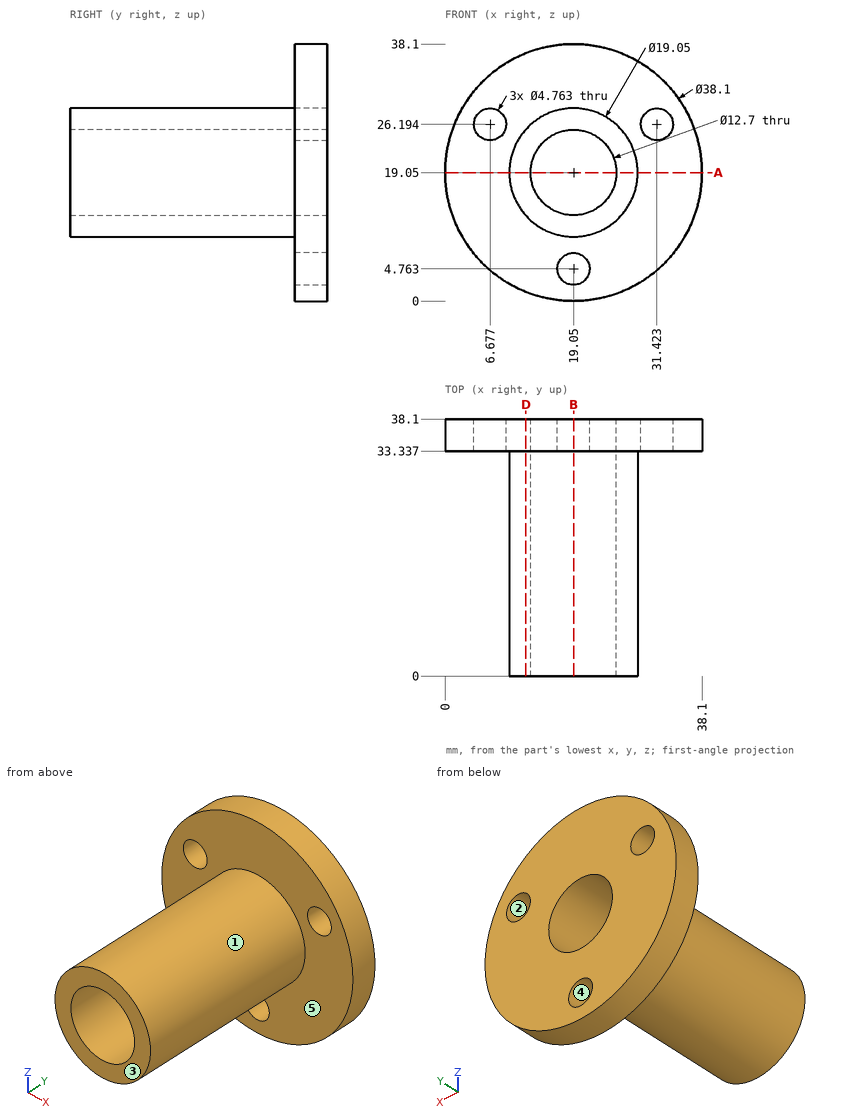
The drawing under review shows one solid part. Ordinate dimensions are in mm from its lowest x, y, z. A direction names the side the tool comes from. Give positions to 0.01 mm unless a question says otherwise; leave off trailing zeros. Write each loop counter-clockwise with the first axis right and the second up, starting at its lowest first coordinate (ties: lowest second). Pieces come first, ordered by that corner, then holes. Notation, with made-up numbers: (-14, 17.25) - (7, 17.25) arc R27 cw to (7, 36.25) - close; hole circle Ø4 at (19.25, -39.5). An arc over 180 degrees is marked (long way). Answer in a Markdown table with one row per item. Add a question column.
1. Draft analysis for pull direction Z (two halves, no side actions). For the marked faces 1, 2 and 3, state which applies: +Z half, -Z half, draft (parallel to the pull), parting line (faces both ways), or undercut.
2. We need section B-B on x = 19.05. Write out the cut boundary in (y, z) (1 decimal), then the cut area to 3 significant figures.
3. Wall thickness on line 1 along X through (y, z) = (14, 19.05) (1 decimal); line 2 along Y through (x, z) = (34, 18.5): over which ranges is each line inside the solid? List them lowest first. Write a range as [from, to].
4. Insertion check: P1, Ø5.5, axis at x = 31.42, z = 26.19, coming from the -Y side; P2, Ø10, axis at x = 6.5, y = 10.5, coming from the +Z side (1 decimal); P3, Ø3, axis at x = 26, y = 23, coming from the +Z side; P4, Ø8, axis at x = 11, z = 16, coming from the -Y side. Each pin has a flat end and moves straight along its axis. Give the tip position at first contact, or say it passes through.
5. We need section A-A on z = 19.05. Write out the cut boundary in (x, y) (1 decimal).
6. We need section D-D on x = 12. Write out the cut boundary in (y, z) (1 decimal).
7. Tool access review of the marked faces 4 and 5: name each direction out of +Z, -Z, +X, -X, +Y, -Y from which nothing blocks a thin tool from reaching the whole face with its end or side.
Ans:
| question | item | result |
|---|---|---|
| 1 | face 1 | parting line |
| 1 | face 2 | undercut |
| 1 | face 3 | draft |
| 2 | outline | (0, 9.5) - (33.3, 9.5) - (33.3, 7.1) - (38.1, 7.1) - (38.1, 12.7) - (0, 12.7) - close; (0, 25.4) - (38.1, 25.4) - (38.1, 38.1) - (33.3, 38.1) - (33.3, 28.6) - (0, 28.6) - close; (33.3, 0) - (38.1, 0) - (38.1, 2.4) - (33.3, 2.4) - close |
| 2 | area | 310 mm^2 |
| 3 | line 1 | x = [9.5, 12.7], [25.4, 28.6] |
| 3 | line 2 | y = [33.34, 38.1] |
| 4 | P1 | stops at y = 33.34 |
| 4 | P2 | stops at z = 24.9 |
| 4 | P3 | stops at z = 26.86 |
| 4 | P4 | stops at y = 0 |
| 5 | outline | (0, 33.3) - (9.5, 33.3) - (9.5, 0) - (12.7, 0) - (12.7, 38.1) - (0, 38.1) - close; (25.4, 0) - (28.6, 0) - (28.6, 33.3) - (38.1, 33.3) - (38.1, 38.1) - (25.4, 38.1) - close |
| 6 | outline | (0, 12.6) - (33.3, 12.6) - (33.3, 1.4) - (38.1, 1.4) - (38.1, 36.7) - (33.3, 36.7) - (33.3, 25.5) - (0, 25.5) - close |
| 7 | face 4 | +Y, -Y |
| 7 | face 5 | -Y |
